Geometry check sheet. Reference: the model listing, model coordinates, mm. A direction names the side the tool comes from. Coordinates: 2 decimals unless noted, no trailing zeros. Loops run counter-clockwise (first coordinate to the right, second up) from the corner with the lowest first, then second, coordinate; pieces in that order, holes last. Notation, with made-up numbers: (71, 52) -> (97, 52) arc R18 ccw to (97, 73) -> close; hole circle Ø9 at (12, 4.25). An arc over 180 degrees is marked (long way). Answer as a JSON object with one key per item and string values.
from build123d import *

# Parameters (mm, degrees)
F2_SIZE = 0.508
F3_R    = 0.508


with BuildPart() as f1:
    # F0 (on Front) → F1 (revolve)
    with BuildSketch(Plane.XZ):
        Polygon((0, 22.225), (0, 5.405244), (5.405244, 0), (9.525, 0), (9.525, 9.525), (3.175, 9.525), (3.175, 22.225), align=None)
    revolve(axis=Axis((0, 0, 17.601646), (0, 0, -1)))

    # F2
    f2_edges = [f1.edges().sort_by_distance(p)[0] for p in [
        (-3.175, 0, 22.225),
    ]]
    chamfer(f2_edges, length=F2_SIZE)

    # F3
    f3_edges = [f1.edges().sort_by_distance(p)[0] for p in [
        (-9.525, 0, 9.525),
        (-3.175, 0, 9.525),
        (-9.525, 0, 0),
    ]]
    fillet(f3_edges, radius=F3_R)


solid = f1.part
1. Section check C-C, the plane z = 8. Record the boundary of the cut face in (x, y) (3 decimals), then the cut area to 3 significant figures.
Evaluation:
{"outline": "circle Ø19.05 at (0, 0)", "area": "285 mm^2"}
2. Tool access check on faces 4 (the face through (-7.559, 5.796, 4.822)), 5 (the face through (4, 0, 9.525)). Record the directions out of +Z, -Z, +X, -X, +Y, -Y that give a thin tool (end or side, any length) a straight path to the whole face; none if there is none.
Evaluation:
{"face 4": "+Z, -Z", "face 5": "+Z"}
3. Section check A-A, the plane z = 2.75. Record the boundary of the cut face in (x, y) (3 decimals).
Evaluation:
{"outline": "circle Ø19.05 at (0, 0); hole circle Ø5.31 at (0, 0)"}
4. Mould release check, pull along Y, two halves, no side actions. Record for faces 1 (the face through (-0.69, 3.1, 15.96)), 2 (the face through (-0.33, 1.5, 3.87)), 3 (the face through (-4, 4, 0)): released by +Y, released by -Y, zero draft, split by the parting line, or undercut.
Evaluation:
{"face 1": "split by the parting line", "face 2": "undercut", "face 3": "zero draft"}
5. Thickness scan on probe 1 along Z at (x, y) = (-7.25, 2) (3 decimals); probe 2 along X at (y, z) = (-1.25, 2.5); probe 3 along Y at (x, z) = (-5.25, 8.75). Record the ranges inside material, lowest first. Write a range as from..to.
Evaluation:
{"probe 1": "z = 0..9.525", "probe 2": "x = -9.44..-2.62, 2.62..9.44", "probe 3": "y = -7.95..7.95"}
6. Depth check by flat-ended pin: P1, Ø1.5, axis at x = -3, z = 9, coming from the +Y side; P2, Ø6, axis at x = -5, z = 9, coming from the -Y side; P3, Ø2, axis at x = 5, z = 6.5, coming from the +Y side; P4, Ø6, axis at x = 6.5, y = -7.5, coming from the -Z side. Enter the tip coordinate at first touch or a pass-through.
Evaluation:
{"P1": "stops at y = 9.26", "P2": "stops at y = -9.31", "P3": "stops at y = 8.64", "P4": "stops at z = 0"}
7. Section check B-B, the plane z = 17. Record the boundary of the cut face in (x, y) (3 decimals), then the cut area to 3 significant figures.
Evaluation:
{"outline": "circle Ø6.35 at (0, 0)", "area": "31.7 mm^2"}
